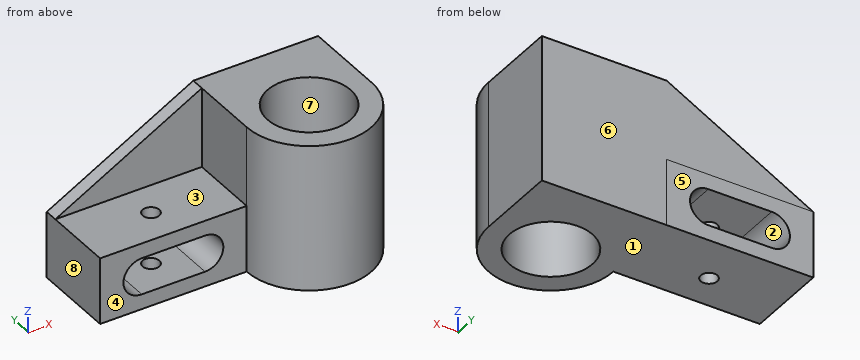
from build123d import *

# Parameters (mm, degrees)
PAD_DEPTH     = 44
SKETCH004_W   = 50
SKETCH004_H   = 40
PAD001_DEPTH  = 88
SKETCH005_R   = 25
HOLE_DEPTH    = 88
POCKET_DEPTH  = 50
SKETCH007_R   = 5
HOLE001_DEPTH = 40
PAD002_DEPTH  = 8


with BuildPart() as part:
    # Sketch → Pad (new body, symmetric)
    with BuildSketch(Plane.XY):
        with BuildLine():
            Line((0, 0), (75, 0))
            Line((75, 0), (75, -50))
            ThreePointArc((0, -50), (37.5, -87.499933), (75, -50))
            Line((0, 0), (0, -50))
        make_face()
    extrude(amount=PAD_DEPTH, both=True)

    # Sketch004 (on Face4 of Pad) → Pad001 (join)
    with BuildSketch(Plane(origin=(0, 0, 0), x_dir=(0, -1, 0), z_dir=(-1, 0, 0))):
        with Locations((24.999986, -24)):
            Rectangle(SKETCH004_W, SKETCH004_H)
    extrude(amount=PAD001_DEPTH)

    # Sketch005 (on Face6 of Pad001) → Hole (cut)
    with BuildSketch(Plane.XY.offset(44)):
        with Locations((37.5, -50)):
            Circle(SKETCH005_R)
    extrude(amount=-HOLE_DEPTH, mode=Mode.SUBTRACT)

    # Sketch006 (on Face10 of Hole) → Pocket (cut)
    with BuildSketch(Plane.XZ.offset(49.999986)):
        with BuildLine():
            ThreePointArc((-25.000028, -35), (-14, -24.000014), (-25, -13))
            Line((-63, -13), (-25, -13))
            ThreePointArc((-63, -13), (-74, -24), (-63, -35))
            Line((-63, -35), (-25.000028, -35))
        make_face()
    extrude(amount=-POCKET_DEPTH, mode=Mode.SUBTRACT)

    # Sketch007 (on Face9 of Pocket) → Hole001 (cut)
    with BuildSketch(Plane.XY.offset(-4)):
        with Locations((-44, -29)):
            Circle(SKETCH007_R)
    extrude(amount=-HOLE001_DEPTH, mode=Mode.SUBTRACT)

    # Sketch008 (on Face1 of Hole001) → Pad002 (join)
    with BuildSketch(Plane(origin=(0, 0, 0), x_dir=(-1, 0, 0), z_dir=(0, 1, 0))):
        Polygon((0, -4), (88, -4), (0, 44), align=None)
    extrude(amount=-PAD002_DEPTH)


solid = part.part
Geometry check sheet. Reference: the model listing, model coordinates, mm. Face numbers are marked on the shaded views. A direction names the side the tool comes from. Round coordinates to 2 decimals unless told otherwise and drop trailing zeros. Loops run counter-clockwise (first coordinate to the right, second up) from the corner with the lowest first, then second, coordinate; pieces in that order, holes last. Notation, with made-up numbers: (51.5, 72.25) - (98.5, 72.25) arc R24 cw to (98.5, 98.25) - close; hole circle Ø3 at (75, -26.5). An arc over 180 degrees is marked (long way). One line per question, with ' | ' between items. Start each with the question number.
1. Scan lines: line 1 (Z direction, x = -35, y = -26); line 2 (Z direction, x = -13, y = -12); line 3 (X direction, y = -49, z = 16.5). Record each from-to range of solid material in increasing order. Write a range as [from, to].
2. Depth check by flat-ended pin: pin 1 (2 mm diameter, centred on x = 54.5, z = -1.5, fed in from -Y); pin 2 (8 mm diameter, centred on x = -44, y = -29, fed in from -Z); pin 3 (4 mm diameter, centred on x = -18, z = -3, fed in from -Y); pin 4 (8 mm diameter, centred on y = -57, z = 29, fed in from +X). Enter the tip coordinate at first touch or a pass-through.
3. Cross-section at D-D on x = 37.5. Record the cut outline in (y, z).
4. Tool access check on the marked faces 1, 2, 3, 4 and 5. Record the directions out of +Z, -Z, +X, -X, +Y, -Y that give a thin tool (end or side, any length) a straight path to the whole face; none if there is none.
5. Cross-section at A-A on z = -24. State how many separate pieces and enclosed holes the cut face has, then the cut area to 3 significant figures.
6. Draft check along X on the marked faces 6, 7 and 8. Enter one of: released by +X, released by -X, zero draft, split by the parting line, or undercut.
7. Cross-section at C-C on y = -10. Record the cut outline in (x, z), then the cut area to 3 significant figures.
Taken from the geometry:
1) line 1: [-44, -35], [-13, -4] | line 2: [-44, -4] | line 3: [0, 12.52], [62.48, 75]
2) pin 1: y = -83.92 | pin 2: through | pin 3: y = -50 | pin 4: x = 74.88
3) outline: (-87.5, -44) - (-75, -44) - (-75, 44) - (-87.5, 44) - close; (-25, -44) - (0, -44) - (0, 44) - (-25, 44) - close
4) face 1: -Z, +X, -X, +Y, -Y | face 2: +Y, -Y | face 3: +Z, -X, -Y | face 4: +Z, -Z, -X, -Y | face 5: +Z, -Z, +X, -X, +Y
5) separate pieces: 2 | enclosed holes: 1 | area: 5,400 mm²
6) face 6: zero draft | face 7: undercut | face 8: released by -X
7) outline: (-88, -44) - (75, -44) - (75, 44) - (0, 44) - (0, -4) - (-88, -4) - close; hole (-63, -35) - (-25, -35) arc R11 ccw to (-25, -13) - (-63, -13) arc R11 ccw to start | area: 8,900 mm²
